Source: CAD feature listing. Evaluate the final solid. Frame: model axes, mm. Face numbers are marked on the shaded views. A direction names the side the tool comes from. Give positions to 0.01 mm unless a question says otherwise; leave off trailing zeros. Loops run counter-clockwise (first coordinate to the right, second up) from the corner with the lowest first, then second, coordinate; pieces in that order, holes last. Notation, with made-up numbers: (12, 32.5) -> (51, 32.5) arc R6 ccw to (51, 37.5) -> close; hole circle Ø7 at (84, -0.5). An arc over 180 degrees is marked (long way). Answer as a JSON object with one key per item and string values. Group by question number.
from build123d import *

# Parameters (mm, degrees)
SM_BASE_FLANGE_1_DEPTH = 2
OTHER_START            = -17.5
OTHER_1_DEPTH          = 35
OTHER_1_2_DEPTH        = 35
OTHER_START_2          = 9.5
OTHER_1_3_DEPTH        = 8
CUT_EXTRUDE_1_DEPTH    = 10
FILLET_1_R             = 3


# Read off the part's stored shape, not the designer's step: 绘制的折弯1
# Sheet-metal steps are written as plain solids
with BuildPart() as part:
    # Sketch 1 → 基体-法兰1 (new body)
    with BuildSketch(Plane(origin=(0, 0, 0), x_dir=(1, 0, 0), z_dir=(0, 1, 0))):
        Polygon((-17.5, -20), (9.5, -20), (9.5, -38), (17.5, -38), (17.5, -20), (17.5, 20), (-17.5, 20), align=None)
    extrude(amount=-SM_BASE_FLANGE_1_DEPTH)

    # Other 1 outline → Other 1 (cut)
    with BuildSketch(Plane.YZ.offset(OTHER_START)):
        with BuildLine():
            ThreePointArc((0, 24), (-0.535898385, 22), (-2, 20.535898384))
            Line((-2, 20.535898384), (-2, -20))
            Line((-2, -20), (0, -20))
            Line((0, -20), (0, 24))
        make_face()
    extrude(amount=OTHER_1_DEPTH, mode=Mode.SUBTRACT)



with BuildPart() as body_2:
    # Other 1 2 outline → Other 1 2 (new body)
    with BuildSketch(Plane.YZ.offset(OTHER_START)):
        with BuildLine():
            ThreePointArc((-3.529524853, 22.056124198), (-3.763094539, 22.014080615), (-4, 22))
            Line((-4, 22), (-43.28761102, 22))
            Line((-43.28761102, 22), (-43.28761102, 20))
            Line((-43.28761102, 20), (-4, 20))
            ThreePointArc((-4, 20), (-3.526189079, 20.02816123), (-3.059049707, 20.112248394))
            Line((-3.059049707, 20.112248394), (-3.529524853, 22.056124198))
        make_face()
    extrude(amount=OTHER_1_2_DEPTH)


with BuildPart() as part_1:
    add(part.part)

    add(body_2.part)  # Other 1 3 merges body 2
    # Other 1 3 outline → Other 1 3 (add)
    with BuildSketch(Plane.YZ.offset(OTHER_START_2)):
        with BuildLine():
            ThreePointArc((-2, 24), (-2.428225479, 22.763260394), (-3.529524853, 22.056124198))
            Line((-3.529524853, 22.056124198), (-3.059049707, 20.112248394))
            ThreePointArc((-3.059049707, 20.112248394), (-2.514346277, 20.286129645), (-2, 20.535898384))
            Line((-2, 20.535898384), (-2, 24))
        make_face()
    extrude(amount=OTHER_1_3_DEPTH)

    # 草图7 → 切除-拉伸1 (cut)
    with BuildSketch(Plane.XZ.offset(2)):
        with BuildLine():
            ThreePointArc((15.1, 35), (14.63137085, 36.13137085), (13.5, 36.6))
            Line((13.5, 36.6), (13.5, 35))
            Line((13.5, 35), (13.5, 33.4))
            ThreePointArc((13.5, 33.4), (14.63137085, 33.86862915), (15.1, 35))
        make_face()
        with BuildLine():
            Line((13.5, 35), (13.5, 36.6))
            ThreePointArc((13.5, 36.6), (11.9, 35), (13.5, 33.4))
            Line((13.5, 33.4), (13.5, 35))
        make_face()
        with BuildLine():
            ThreePointArc((15.1, 27), (14.63137085, 28.13137085), (13.5, 28.6))
            Line((13.5, 28.6), (13.5, 27))
            Line((13.5, 27), (13.5, 25.4))
            ThreePointArc((13.5, 25.4), (14.63137085, 25.86862915), (15.1, 27))
        make_face()
        with BuildLine():
            Line((13.5, 27), (13.5, 28.6))
            ThreePointArc((13.5, 28.6), (11.9, 27), (13.5, 25.4))
            Line((13.5, 25.4), (13.5, 27))
        make_face()
    extrude(amount=-CUT_EXTRUDE_1_DEPTH, mode=Mode.SUBTRACT)

    # 圆角1
    fillet_1_edges = [part_1.edges().sort_by_distance(p)[0] for p in [
        (-17.5, -43.28761102, 21),
        (17.5, -43.28761102, 21),
        (17.5, -1, 38),
        (9.5, -1, 38),
        (-17.5, -3.29428728, 21.084186296),
    ]]
    fillet(fillet_1_edges, radius=FILLET_1_R)


solid = part_1.part
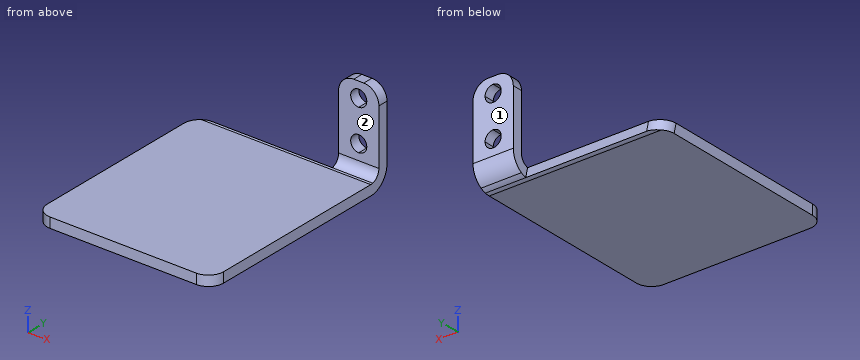
(1) Material intervals for line 1 (Z direction, x = -12, y = -12); line 2 (Y direction, x = 12, z = 33.5); line 3 (Y direction, x = 16, z = 22.75), sorted ascending. Write a range as from..to.
(2) Section query B-B on z = 24.75. Return the cut outline in (x, y), plus the area to 3 significant figures.
(3) Access query for the marked faces 1 and 2. Directions: +Z, -Z, +X, -X, +Y, -Y. A direction counts if a zero-diameter tool reaches every point of the face in a straight line with its end or side. Return the directions, or none.
(4) First-contact query: pin 1 (1.8 mm diameter, centred on y = -2, z = 25, fed in from -X); pin 2 (6.5 mm diameter, centred on x = 15, z = 29, fed in from -Y); pin 3 (6 mm diameter, centred on y = -33, z = 23, fed in from +X); pin 4 (3 mm diameter, centred on x = 6.5, z = 25.5, fed in from -Y). Flat tips, straight axial feed; report the tip coordinate or a pass-through.
(5) Section query A-A on x = 4.5. Return the cut outline in (y, z), plus the area to 3 significant figures.
(6) Section query D-D on x = -15. Return the cut outline in (y, z), plus the area to 3 significant figures.
(7) Section query C-C on y = -32. Return the cut outline in (x, z).
Result:
{
 "1": {"line 1": "20..22", "line 2": "-2..0", "line 3": "-2.44..-0.2"},
 "2": {"outline": "(9.5, -2) -> (17.5, -2) -> (17.5, 0) -> (9.5, 0) -> close", "area": "16.0 mm²"},
 "3": {"face 1": "+Z, -Z, +X, -X, +Y", "face 2": "+Z, +X, -X, -Y"},
 "4": {"pin 1": "x = 9.5", "pin 2": "y = -2", "pin 3": "x = 17.5", "pin 4": "through"},
 "5": {"outline": "(-43.29, 20) -> (-4, 20) arc R4 ccw to (-3.06, 20.11) -> (-3.53, 22.06) arc R2 cw to (-4, 22) -> (-43.29, 22) -> close", "area": "80.0 mm²"},
 "6": {"outline": "(-43.25, 20) -> (-4, 20) arc R4 ccw to (-3.1, 20.1) -> (-3.57, 22.05) arc R2 cw to (-4, 22) -> (-43.25, 22) -> close", "area": "79.8 mm²"},
 "7": {"outline": "(-17.5, 20) -> (17.5, 20) -> (17.5, 22) -> (-17.5, 22) -> close"}
}
